Source: CAD feature listing. Evaluate the final solid. Frame: model axes, mm. A direction names the side the tool comes from. Round coordinates to 2 decimals unless told otherwise and drop trailing zeros. Write each loop counter-clockwise with the first axis right and the second up, starting at its lowest first coordinate (ties: lowest second). Pieces come first, ordered by that corner, then holes.
from build123d import *

# Parameters (mm, degrees)
F0_W     = 1000
F0_H     = 100
F1_DEPTH = 50
F2_W     = 43.5
F2_H     = 93.5
F3_DEPTH = 1000
F4_R     = 5


with BuildPart() as f1:
    # F0 (on Front) → F1 (new body)
    with BuildSketch(Plane.XZ):
        with Locations((-0.774916, 2.339742)):
            Rectangle(F0_W, F0_H)
    extrude(amount=F1_DEPTH)

    # F2 (on face) → F3 (cut, through all)
    with BuildSketch(Plane.YZ.offset(499.225084)):
        with Locations((-25, 2.339742)):
            Rectangle(F2_W, F2_H)
    extrude(amount=-F3_DEPTH, mode=Mode.SUBTRACT)

    # F4
    f4_edges = [f1.edges().sort_by_distance(p)[0] for p in [
        (-0.774916, -50, 52.339742),
        (-0.774916, 0, 52.339742),
        (-0.774916, -50, -47.660258),
        (-0.774916, 0, -47.660258),
    ]]
    fillet(f4_edges, radius=F4_R)


solid = f1.part
1) Section query C-C on z = -27. Return the cut outline in (x, y), then the cut area to 3 significant figures.
Taken from the geometry:
outline: (-500.77, -50) - (499.23, -50) - (499.23, -46.75) - (-500.77, -46.75) - close; (-500.77, -3.25) - (499.23, -3.25) - (499.23, 0) - (-500.77, 0) - close
area: 6,500 mm2
2) Reachability of faces 4 (the face through (499.225, -47, 2)), 5 (the face through (6, -25, -44.41)) from +Z, -Z, +X, -X, +Y, -Y: full face, straight path, thin tool, end or side. Return the list, or none.
Taken from the geometry:
face 4: +Z, -Z, +X, +Y, -Y
face 5: +X, -X
3) Section query B-B on x = 26. Return the cut outline in (y, z), then the cut area to 3 significant figures.
Taken from the geometry:
outline: (-50, -42.66) arc R5 ccw to (-45, -47.66) - (-5, -47.66) arc R5 ccw to (0, -42.66) - (0, 47.34) arc R5 ccw to (-5, 52.34) - (-45, 52.34) arc R5 ccw to (-50, 47.34) - close; hole (-46.75, -44.41) - (-3.25, -44.41) - (-3.25, 49.09) - (-46.75, 49.09) - close
area: 911 mm2
4) Section query A-A on y = -29.5. Return the cut outline in (x, z), then the cut area to 3 significant figures.
Taken from the geometry:
outline: (-500.77, -47.66) - (499.23, -47.66) - (499.23, -44.41) - (-500.77, -44.41) - close; (-500.77, 49.09) - (499.23, 49.09) - (499.23, 52.34) - (-500.77, 52.34) - close
area: 6,500 mm2
5) Pull-direction query (Z, two-part tool) for faces 1 (the face through (6, -3.25, 2)), 2 (the face through (-8, -25, -47.66)), 3 (the face through (-8, 0, 3)); classes: released by +Z, released by -Z, zero draft, split by the parting line, or undercut.
Taken from the geometry:
face 1: undercut
face 2: released by -Z
face 3: zero draft
6) Material intervals for line 1 (Y direction, x = -311, z = -40); line 2 (Z direction, x = -429, y = -45); line 3 (Z direction, x = 252, y = -4), sorted ascending.
Taken from the geometry:
line 1: y = -50 to -46.75, -3.25 to 0
line 2: z = -47.66 to -44.41, 49.09 to 52.34
line 3: z = -47.56 to -44.41, 49.09 to 52.24
